Read the model definition and answer for the solid it produces. Units are mm, in the model's axes. A direction names the side the tool comes from. Round coordinates to 2 decimals unless told otherwise and drop trailing zeros. Write each loop counter-clockwise with the first axis right and the second up, starting at its lowest first coordinate (ties: lowest second). Pieces come first, ordered by that corner, then holes. Notation, with made-up numbers: (37.5, 7) - (91.5, 7) arc R19 ccw to (91.5, 28) - close; hole circle Ø6 at (85.25, 32). An arc over 180 degrees is marked (long way). One line per item, written item: value. Start each with the question number.
(1) A cutting plane is placed at A-A, the plane y = 63.5. Determine the outline of the cut face in (x, z) (3 decimals), plus the area to 3 significant figures.
(2) For faces 1 (the face through (28, 10, -444.5)), 2 (the face through (57, 12.7, -45)), 3 (the face through (51, 6, 342.9)), determine the directions among +Z, -Z, +X, -X, +Y, -Y from which every point of the face is accessible in a straight line to the end or side of a thin tool.
(3) A cutting plane is placed at C-C, the plane z = -406.4. Determine the outline of the cut face in (x, y) (3 decimals).
(4) A cutting plane is placed at D-D, the plane z = 58. Determine the outline of the cut face in (x, y) (3 decimals), plus the area to 3 significant figures.
(5) Flat-ended cylindrical pins translate along their axes: pin 1 Ø6 at (x, z) = (38, -185) entering from +Y; pin 2 Ø12 at (y, z) = (60.5, 98) entering from +X; pin 3 Ø5 at (y, z) = (61.5, -85.5) entering from -X; pin 4 Ø17 at (x, z) = (50.8, -406.4) entering from +Y. Find the tip coordinate at first contact, or state that the pin passes through.
(6) The mould has two halves that part along X. Classify faces 4 (the face through (12.7, 56, -6)), 5 (the face through (52, 0, 6)), 6 (the face through (52.04, 6.439, -396.956)): +X half, -X half, draft (parallel to the pull), parting line (faces both ways), or undercut.
(7) Find the intervals of material crossed by L1, parallel to Z at x = 50.8, y = 3 (3 decimals); L2, parallel to X at y = 5, z = -406; L3, parallel to Y at x = 44, z = 83, in increasing order.
(8) A cutting plane is placed at B-B, the plane x = 50.8. Determine the outline of the cut face in (y, z) (3 decimals).
from build123d import *

# Parameters (mm, degrees)
BOSS_EXTRUDE1_DEPTH             = 444.5
CUT_EXTRUDE1_REACH              = 103.6
CUT_EXTRUDE2_REACH              = 103.6
F_3_4_0_75_DIAMETER_HOLE1_D     = 19.05
F_3_4_0_75_DIAMETER_HOLE1_DEPTH = 50.8
F_3_4_0_75_DIAMETER_HOLE1_TIP   = 5.723197396


with BuildPart() as part:
    # Sketch1 → Boss-Extrude1 (new body, symmetric)
    with BuildSketch(Plane.XY):
        with BuildLine():
            Line((0, 0), (0, 101.6))
            Line((0, 101.6), (3.18008, 101.6))
            ThreePointArc((3.18008, 101.6), (9.911679988, 98.811679988), (12.7, 92.08008))
            Line((12.7, 92.08008), (12.7, 22.225))
            ThreePointArc((12.7, 22.225), (15.489807909, 15.489807909), (22.225, 12.7))
            Line((22.225, 12.7), (92.08008, 12.7))
            ThreePointArc((92.08008, 12.7), (98.811679988, 9.911679988), (101.6, 3.18008))
            Line((101.6, 3.18008), (101.6, 0))
            Line((101.6, 0), (0, 0))
        make_face()
    extrude(amount=BOSS_EXTRUDE1_DEPTH, both=True)

    # Sketch2 → Cut-Extrude1 (cut, up to next)
    with BuildSketch(Plane.XZ, mode=Mode.PRIVATE) as cut_extrude1_sk1:
        Polygon((88.9, 342.9), (12.7, 342.9), (12.7, 444.5), (101.6, 444.5), (101.6, 342.9), (101.6, 330.2), align=None)
    cut_extrude1_tool1 = extrude(cut_extrude1_sk1.sketch, amount=-CUT_EXTRUDE1_REACH, mode=Mode.PRIVATE) & part.part
    add(cut_extrude1_tool1.solids().sort_by_distance((57.5059, 0, 393.212979))[0], mode=Mode.SUBTRACT)

    # Sketch3 → Cut-Extrude2 (cut, up to next)
    with BuildSketch(Plane.ZY, mode=Mode.PRIVATE) as cut_extrude2_sk1:
        with BuildLine():
            Line((419.1, 53.975), (400.05, 53.975))
            ThreePointArc((400.05, 53.975), (390.525, 63.5), (400.05, 73.025))
            Line((400.05, 73.025), (419.1, 73.025))
            ThreePointArc((419.1, 73.025), (428.625, 63.5), (419.1, 53.975))
        make_face()
    cut_extrude2_tool1 = extrude(cut_extrude2_sk1.sketch, amount=-CUT_EXTRUDE2_REACH, mode=Mode.PRIVATE) & part.part
    add(cut_extrude2_tool1.solids().sort_by_distance((0, 63.5, 409.575))[0], mode=Mode.SUBTRACT)

    # 3/4 (0.75) Diameter Hole1
    with Locations(Plane.XZ):
        with Locations((50.8, -406.4)):
            Hole(F_3_4_0_75_DIAMETER_HOLE1_D / 2, depth=F_3_4_0_75_DIAMETER_HOLE1_DEPTH)
            with Locations((0, 0, -(F_3_4_0_75_DIAMETER_HOLE1_DEPTH + F_3_4_0_75_DIAMETER_HOLE1_TIP / 2))):  # 118° drill point
                Cone(0, F_3_4_0_75_DIAMETER_HOLE1_D / 2, F_3_4_0_75_DIAMETER_HOLE1_TIP, mode=Mode.SUBTRACT)


solid = part.part
Here are the results:
1. outline: (0, -444.5) - (12.7, -444.5) - (12.7, 390.525) - (0, 390.525) - close; (0, 428.625) - (12.7, 428.625) - (12.7, 444.5) - (0, 444.5) - close
1. area: 10,800 mm²
2. face 1: -Z, +X, -X, +Y, -Y
2. face 2: +Z, -Z, +X, +Y
2. face 3: +Z, +X, +Y, -Y
3. outline: (0, 0) - (41.275, 0) - (41.275, 12.7) - (22.225, 12.7) arc R9.525 cw to (12.7, 22.225) - (12.7, 92.08) arc R9.52 ccw to (3.18, 101.6) - (0, 101.6) - close; (60.325, 0) - (101.6, 0) - (101.6, 3.18) arc R9.52 ccw to (92.08, 12.7) - (60.325, 12.7) - close
4. outline: (0, 0) - (101.6, 0) - (101.6, 3.18) arc R9.52 ccw to (92.08, 12.7) - (22.225, 12.7) arc R9.525 cw to (12.7, 22.225) - (12.7, 92.08) arc R9.52 ccw to (3.18, 101.6) - (0, 101.6) - close
4. area: 2,400 mm²
5. pin 1: y = 12.7
5. pin 2: x = 12.7
5. pin 3: x = 0
5. pin 4: through
6. face 4: +X half
6. face 5: draft
6. face 6: undercut
7. L1: -444.5 to -415.925, -396.875 to 342.9
7. L2: 0 to 41.28, 60.32 to 101.42
7. L3: 0 to 12.7
8. outline: (0, -444.5) - (12.7, -444.5) - (12.7, -415.925) - (0, -415.925) - close; (0, -396.875) - (12.7, -396.875) - (12.7, 342.9) - (0, 342.9) - close
